```python
from build123d import *

# Parameters (mm, degrees)
SKETCH1_W                              = 101.6
SKETCH1_H                              = 127
BOSS_EXTRUDE1_DEPTH                    = 12.7
SKETCH4_R                              = 6.35
CUT_EXTRUDE9_DEPTH                     = 164.134453749
CBORE_FOR_M5_HEX_HEAD_BOLT1_AT_2_COUNT = 2
CBORE_FOR_M5_HEX_HEAD_BOLT1_AT_2_PITCH = 18.0086
CBORE_FOR_M5_HEX_HEAD_BOLT1_AT_3_COUNT = 2
CBORE_FOR_M5_HEX_HEAD_BOLT1_AT_3_PITCH = 25.461925967
CBORE_FOR_M5_HEX_HEAD_BOLT1_AT_4_COUNT = 2
CBORE_FOR_M5_HEX_HEAD_BOLT1_AT_4_PITCH = 18


with BuildPart() as part:
    # Sketch1 → Boss-Extrude1 (new body)
    with BuildSketch(Plane.XY):
        with Locations((50.8, 63.5)):
            Rectangle(SKETCH1_W, SKETCH1_H)
    extrude(amount=BOSS_EXTRUDE1_DEPTH)

    # Sketch4 → Cut-Extrude9 (cut, through all)
    with BuildSketch(Plane.XY.offset(12.7)):
        with Locations((12.7, 114.3)):
            Circle(SKETCH4_R)
        with Locations((12.7, 25.4)):
            Circle(SKETCH4_R)
        with Locations(Location((88.9, 25.4, 0), (0, 0, 180))):
            Circle(SKETCH4_R)
        with Locations(Location((88.9, 114.3, 0), (0, 0, 180))):
            Circle(SKETCH4_R)
    extrude(amount=-CUT_EXTRUDE9_DEPTH, mode=Mode.SUBTRACT)

    # Sketch8 → CBORE for M5 Hex Head Bolt1 (revolve, cut)
    with BuildSketch(Plane(origin=(41.7957, 72.5, 12.7), x_dir=(0, -1, 0), z_dir=(1, 0, 0))):
        Polygon((0, 0), (0, 12.7), (2.75, 12.7), (2.75, 3.58), (6.12, 3.58), (6.12, 0.025), (6.145, 0), align=None)
    cbore_for_m5_hex_head_bolt1 = revolve(axis=Axis((41.7957, 72.5, 19.05), (0, 0, -1)), mode=Mode.SUBTRACT)

    # CBORE for M5 Hex Head Bolt1 at 2: CBORE for M5 Hex Head Bolt1 ×2
    with Locations(*[(i * CBORE_FOR_M5_HEX_HEAD_BOLT1_AT_2_PITCH, 0, 0) for i in range(1, CBORE_FOR_M5_HEX_HEAD_BOLT1_AT_2_COUNT)]):
        add(cbore_for_m5_hex_head_bolt1, mode=Mode.SUBTRACT)

    # CBORE for M5 Hex Head Bolt1 at 3: CBORE for M5 Hex Head Bolt1 ×2
    with Locations(*[Vector(0.7072756406246394, -0.7069378814146302, 0) * (i * CBORE_FOR_M5_HEX_HEAD_BOLT1_AT_3_PITCH) for i in range(1, CBORE_FOR_M5_HEX_HEAD_BOLT1_AT_3_COUNT)]):
        add(cbore_for_m5_hex_head_bolt1, mode=Mode.SUBTRACT)

    # CBORE for M5 Hex Head Bolt1 at 4: CBORE for M5 Hex Head Bolt1 ×2
    with Locations(*[(0, -i * CBORE_FOR_M5_HEX_HEAD_BOLT1_AT_4_PITCH, 0) for i in range(1, CBORE_FOR_M5_HEX_HEAD_BOLT1_AT_4_COUNT)]):
        add(cbore_for_m5_hex_head_bolt1, mode=Mode.SUBTRACT)


solid = part.part
```
Geometry: final body of the model. Coordinates: model frame, mm. A direction names the side the tool comes from. Give positions to 0.01 mm unless a question says otherwise; leave off trailing zeros. Loops run counter-clockwise (first coordinate to the right, second up) from the corner with the lowest first, then second, coordinate; pieces in that order, holes last. Notation, with made-up numbers: (83, 75.25) - (141, 75.25) arc R24 ccw to (141, 113.25) - close; hole circle Ø11 at (81.5, 56). An arc over 180 degrees is marked (long way). Answer as CSV lines item,"result". Start each with the question number.
(1) Section query B-B (z = 5.5). Give the number of separate pieces and of enclosed holes in the cut face, and give its area (3 significant figures).
(2) Section query A-A (y = 54.5). Output: boundary loops of the cut face in (x, z) (3 decimals), and give its area (3 significant figures).
(3) Ray query, line 1 along Y through (x, z) = (88.9, 7.5); line 2 along X through (y, z) = (54.5, 3.25); line 3 along X through (y, z) = (26, 8). Return the intervals inside material, ascending. Write a range as [from, to].
(4) Section query C-C (y = 25.4). Output: boundary loops of the cut face in (x, z).
(5) Mould query, pull axis X, two halves, no side actions, for faces 3 (the face through (44.4, 55.8, 9.12)), 4 (the face through (101.6, 63, 6)), 5 (the face through (61.1, 75.1, 9.12)), 6 (the face through (50, 64, 0)). Classes: +X half, -X half, draft (parallel to the pull), parting line (faces both ways), or undercut.
(6) Pin query (flat end, axial travel): P1, Ø7, axis at x = 41.8, y = 54.5, coming from the +Z side; P2, Ø3.5, axis at x = 59.8, y = 54.5, coming from the +Z side. Return the tip coordinate at first contact, or that it passes through.
(7) Reachability of faces 1 (the face through (62.4, 55.8, 9.12)), 2 (the face through (7.66, 21.54, 6.44)) from +Z, -Z, +X, -X, +Y, -Y: full face, straight path, thin tool, end or side. Return the list, or none.
Worked answers:
1,separate pieces,"1"
1,enclosed holes,"8"
1,area,"12,300 mm^2"
2,outline,"(0, 0) - (39.046, 0) - (39.046, 9.12) - (35.676, 9.12) - (35.676, 12.675) - (35.651, 12.7) - (0, 12.7) - close; (44.546, 0) - (57.054, 0) - (57.054, 9.12) - (53.684, 9.12) - (53.684, 12.675) - (53.659, 12.7) - (47.941, 12.7) - (47.916, 12.675) - (47.916, 9.12) - (44.546, 9.12) - close; (62.554, 0) - (101.6, 0) - (101.6, 12.7) - (65.949, 12.7) - (65.924, 12.675) - (65.924, 9.12) - (62.554, 9.12) - close"
2,area,"1,100 mm^2"
3,line 1,"y = [0, 19.05], [31.75, 107.95], [120.65, 127]"
3,line 2,"x = [0, 39.05], [44.55, 57.05], [62.55, 101.6]"
3,line 3,"x = [0, 6.38], [19.02, 82.58], [95.22, 101.6]"
4,outline,"(0, 0) - (6.35, 0) - (6.35, 12.7) - (0, 12.7) - close; (19.05, 0) - (82.55, 0) - (82.55, 12.7) - (19.05, 12.7) - close; (95.25, 0) - (101.6, 0) - (101.6, 12.7) - (95.25, 12.7) - close"
5,face 3,"undercut"
5,face 4,"+X half"
5,face 5,"undercut"
5,face 6,"draft"
6,P1,"stops at z = 9.12"
6,P2,"passes through"
7,face 1,"+Z"
7,face 2,"+Z, -Z"
